Autodesk Inventor part; units mm, degrees
ref_plane "Arbeitsebene1" through (-17, 4, 20) normal (1, 0, 0) x (0, -1, 0)
ref_plane "YZ Plane" through (0, 0, 0) normal (1, 0, 0) x (0, 1, 0)
ref_plane "XZ Plane" through (0, 0, 0) normal (0, 1, 0) x (-1, 0, 0)
sketch "Sketch1" plane through (0, 0, 0) normal (0, 1, 0) x (-1, 0, 0)
  line L0 (20, 20) -> (-20, 20)
  line L1 (-20, 20) -> (-20, -20)
  line L2 (-20, -20) -> (20, -20)
  line L3 (20, -20) -> (20, 20)
  circle A0 centre (12.5, 12.5) radius 4.25
  circle A1 centre (12.5, -12.5) radius 4.25
  circle A2 centre (-12.5, -12.5) radius 4.25
  circle A3 centre (-12.5, 12.5) radius 4.25
  line L4 (20, 0) -> (-20, 0) construction
  line L5 (0, 20) -> (0, -20) construction
  point P0 (0, 0)
  dimension "d0" = 40
  dimension "d1" = 40
  dimension "d2" = 8.5
  dimension "d3" = 25
  dimension "d4" = 25
extrude "Extrusion2" add sketch "Sketch1" along normal blind 2
sketch "Sketch2" plane through (0, 0, 0) normal (0, -1, 0) x (1, 0, 0)
  line L0 (20, 20) -> (20, -20)
  line L1 (-20, 20) -> (20, 20)
  line L2 (-20, -20) -> (-20, 20)
  line L3 (20, -20) -> (-20, -20)
  point P0 (0, 0)
extrude "Extrusion3" add sketch "Sketch2" along normal blind 0.6
sketch "Sketch3" plane through (0, 2, 0) normal (0, 1, 0) x (1, 0, 0)
  line L0 (-20, 20) -> (-20, -20)
  line L1 (-20, -20) -> (20, -20)
  line L2 (20, -20) -> (20, 20)
  line L3 (20, 20) -> (-20, 20)
  point P0 (0, 0)
extrude "Extrusion4" add sketch "Sketch3" along normal blind 2
sketch "Sketch4" plane through (0, 4, 0) normal (0, 1, 0) x (1, 0, 0)
  circle A0 centre (-8, -7.5305) radius 1.4
  circle A1 centre (-8, 7.5305) radius 1.4
  line L0 (-20, -20) -> (-20, 20)
  line L1 (-20, 0) -> (20, 0) construction
  line L2 (20, 20) -> (20, -20)
  point P0 (0, 0)
  dimension "d13" = 15.061
  dimension "d14" = 2.8
  dimension "d15" = 12
extrude "Extrusion5" add sketch "Sketch4" along normal blind 5
chamfer "Chamfer1" distance 0.5 angle 45 2 edges at (-9.4, 4, 7.5305) (-9.4, 4, -7.5305)
fillet "Fillet1" radius 3 4 edges at (-20, 1.7, 20) (-20, 1.7, -20) (20, 1.7, 20) (20, 1.7, -20)
ref_plane "Arbeitsebene1" through (-17, 4, 20) normal (1, 0, 0) x (0, -1, 0)
sketch "Skizze5" plane through (-17, 4, 20) normal (1, 0, 0) x (0, -1, 0)
  line L0 (0, 0) -> (4.6, 0) construction
  line L1 (0, 0) -> (0, 3) construction
  line L2 (0.7, 0) -> (3.5, 0) construction
  line L3 (6.1491, 20) -> (-1.642, 20) construction
  line L4 (0, 40) -> (4.6, 40) construction
  line L5 (0.7, 40) -> (3.5, 40) construction
  line L6 (2.3, 0) -> (2.3, 4.6722) construction
  ellipse E0 centre (2.3, 0) end of major axis (3.5, 0) minor radius 1
  line L7 (1.1, 0) -> (3.5, 0)
  line L8 (0, 40) -> (4.6, 40) construction
  line L9 (0.7, 40) -> (3.5, 40) construction
  ellipse E1 centre (2.3, 40) end of major axis (3.5, 40) minor radius 1
  line L10 (1.1, 40) -> (3.5, 40)
  point P0 (4, 20)
  point P1 (2.3, 1)
  dimension "d22" = 2.3
  dimension "d23" = 1.2
  dimension "d28" = 1
extrude "Extrusion7" cut sketch "Skizze5" along normal blind 37 and the other way blind 5 contours L7 E0 | E1 L10 picked at (2.3176, 0.333) picked at (2.2824, 39.667)
properties part number "IMU_mount_baseplate"
Read the model definition and answer for the solid it produces. Units are mm, in the model's axes. A direction names the side the tool comes from. Round coordinates to 2 decimals unless told otherwise and drop trailing zeros. Write each loop counter-clockwise with the first axis right and the second up, starting at its lowest first coordinate (ties: lowest second). Pieces come first, ordered by that corner, then holes.
Q1. Flat-ended cylindrical pins translate along their axes: P1, Ø7, axis at x = 12.5, z = 12.5, coming from the +Y side; P2, Ø7, axis at x = -12, z = -10.5, coming from the +Y side; P3, Ø9.5, axis at x = -10.5, z = 10.5, coming from the +Y side. Find the tip coordinate at first contact, or state that the pin passes through.
Values:
P1: stops at y = 4
P2: stops at y = 4.42
P3: stops at y = 9
Q2. Find section B-B on y = 5.25. Determine the outline of the cut face in (x, z).
Values:
outline: circle Ø2.8 at (-8, -7.53); circle Ø2.8 at (-8, 7.53)
Q3. Find section A-A on z = 12.5. Determine the outline of the cut face in (x, y).
Values:
outline: (-20, -0.6) - (20, -0.6) - (20, 4) - (-20, 4) - close; hole (-16.75, 0) - (-8.25, 0) - (-8.25, 2) - (-16.75, 2) - close; hole (8.25, 0) - (16.75, 0) - (16.75, 2) - (8.25, 2) - close
Q4. Find section D-D on z = 4. Determine the outline of the cut face in (x, y).
Values:
outline: (-20, -0.6) - (20, -0.6) - (20, 4) - (-20, 4) - close
Q5. The mould has two halves that part along Y. Classify faces 1 (the face through (-13, 2, 12)), 2 (the face through (-8, 9, 8)), 3 (the face through (20, 2, 0)): released by +Y, released by -Y, zero draft, split by the parting line, or undercut.
Values:
face 1: undercut
face 2: released by +Y
face 3: zero draft
Q6. A tool of negligible diameter and unlimited length cuts with its end or side. For faces 4 (the face through (-13, 2, -13)), 5 (the face through (-0.2, 3.4, 20)), from which of +Z, -Z, +X, -X, +Y, -Y can it reach the whole face along a straight path? Write none if from no direction.
Values:
face 4: none
face 5: +Z, +X, -X, +Y, -Y
Q7. Find section C-C on x = -14.5. State how many separate pieces and enclosed holes the cut face has, and give its area (3 significant figures).
Values:
separate pieces: 1
enclosed holes: 2
area: 150 mm2
Q8. Straight lines are drawn through the part: line 1 (Y direction, x = 10.5, z = 14); line 2 (Z direction, x = -16, y = 1); line 3 (Z direction, x = 12.5, y = 0.8). For each, find the intervals that lie inside material, in ascending order.
Values:
line 1: y = -0.6 to 0, 2 to 4
line 2: z = -19.19 to -14.91, -10.09 to 10.09, 14.91 to 19.19
line 3: z = -19.34 to -16.75, -8.25 to 8.25, 16.75 to 19.34
